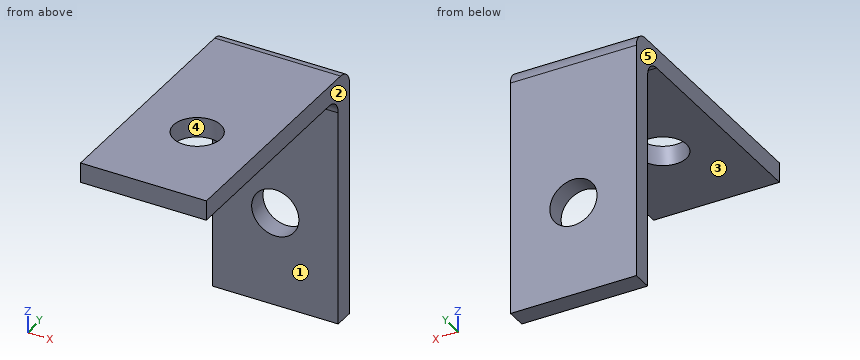
```python
from build123d import *

# Parameters (mm, degrees)
CROQUIS1_W              = 12.7
CROQUIS1_H              = 25.4
SALIENTE_EXTRUIR1_DEPTH = 2
CROQUIS2_W              = 12.7
CROQUIS2_H              = 2
SALIENTE_EXTRUIR2_DEPTH = 23.368
REDONDEO1_R             = 1.5875
CROQUIS3_R              = 2.38125
CORTAR_EXTRUIR1_DEPTH   = 26.368
CROQUIS4_R              = 2.38125
CORTAR_EXTRUIR2_DEPTH   = 2.54


with BuildPart() as part:
    # Croquis1 → Saliente-Extruir1 (new body)
    with BuildSketch(Plane(origin=(0, 0, 0), x_dir=(1, 0, 0), z_dir=(0, 1, 0))):
        Rectangle(CROQUIS1_W, CROQUIS1_H)
    extrude(amount=SALIENTE_EXTRUIR1_DEPTH)

    # Croquis2 → Saliente-Extruir2 (add)
    with BuildSketch(Plane.XZ):
        with Locations((0, 11.7)):
            Rectangle(CROQUIS2_W, CROQUIS2_H)
    extrude(amount=SALIENTE_EXTRUIR2_DEPTH)

    # Redondeo1
    redondeo1_edges = [part.edges().sort_by_distance(p)[0] for p in [
        (0, 2, 12.7),
        (0, 0, 10.7),
    ]]
    fillet(redondeo1_edges, radius=REDONDEO1_R)

    # Croquis3 → Cortar-Extruir1 (cut, through all)
    with BuildSketch(Plane(origin=(0, 2, 0), x_dir=(1, 0, 0), z_dir=(0, 1, 0))):
        with Locations((0, 3.175)):
            Circle(CROQUIS3_R)
    extrude(amount=-CORTAR_EXTRUIR1_DEPTH, mode=Mode.SUBTRACT)

    # Croquis4 → Cortar-Extruir2 (cut)
    with BuildSketch(Plane.XY.offset(12.7)):
        with Locations((0, -13.843)):
            Circle(CROQUIS4_R)
    extrude(amount=-CORTAR_EXTRUIR2_DEPTH, mode=Mode.SUBTRACT)


solid = part.part
```
Part model, mm, in its own coordinate system. Face numbers are marked on the shaded views. A direction names the side the tool comes from. Coordinates: 2 decimals unless noted, no trailing zeros. Order: outer loops, then holes, each group sorted by start corner. A loop starts at its lowest first (then second) coordinate and runs counter-clockwise, first axis right, second up. Notation, with made-up numbers: (69.5, -29) -> (106.5, -29) arc R29 ccw to (106.5, 5) -> close; hole circle Ø6 at (-11.5, -17). An arc over 180 degrees is marked (long way). Put each result on its own line as item: value. Start each with the question number.
(1) Band-saw the part on D-D (z = 2). Give the cut face in (x, y), then the cut area to 3 significant figures.
(2) Which spindle directions (+Z, -Z, +X, -X, +Y, -Y) get a long thin tool onto all of the face, cutting with end or side? Do the marked faces 1 and 2. Say none if no direction does.
(3) Mould opens along X. For the marked faces 3, 4 and 5 say: pulls with the +X half, pulls with the -X half, needs draft (parallel to the pull), parting line crosses it, or undercut.
(4) Band-saw the part on B-B (x = 4). Give the cut face in (y, z) (1 decimal).
(5) Pin check, flat tips, straight feed: pin 1 Ø6.5 at (x, z) = (-1.5, 3.5) entering from -Y; pin 2 Ø6 at (x, y) = (1, -13.5) entering from -Z. Stop position of each tip, or through.
(6) Band-saw the part on C-C (y = -5.25). Give the cut face in (x, z).
(7) Probe line 1 along Z through (x, y) = (-1.5, -18.75); line 2 along Y through (x, z) = (-1.75, 6.5); line 3 along Z through (x, y) = (0, 1.4). List the from-to ranges inside material, lowest first. Write a range as [from, to].
(8) Band-saw the part on A-A (x = 0). Give the cut face in (y, z) (1 decimal).
Determined:
1. outline: (-6.35, 0) -> (6.35, 0) -> (6.35, 2) -> (-6.35, 2) -> close
1. area: 25.4 mm²
2. face 1: -Z, +X, -X, -Y
2. face 2: +Z, -Z, +X, +Y, -Y
3. face 3: needs draft
3. face 4: undercut
3. face 5: pulls with the -X half
4. outline: (-23.4, 10.7) -> (-1.6, 10.7) arc R1.6 cw to (0, 9.1) -> (0, -12.7) -> (2, -12.7) -> (2, 11.1) arc R1.6 ccw to (0.4, 12.7) -> (-23.4, 12.7) -> close
5. pin 1: stops at y = 0
5. pin 2: stops at z = 10.7
6. outline: (-6.35, 10.7) -> (6.35, 10.7) -> (6.35, 12.7) -> (-6.35, 12.7) -> close
7. line 1: z = [10.7, 12.7]
7. line 2: y = [0, 2]
7. line 3: z = [-12.7, -5.56], [-0.79, 12.36]
8. outline: (-23.4, 10.7) -> (-16.2, 10.7) -> (-16.2, 12.7) -> (-23.4, 12.7) -> close; (-11.5, 10.7) -> (-1.6, 10.7) arc R1.6 cw to (0, 9.1) -> (0, -0.8) -> (2, -0.8) -> (2, 11.1) arc R1.6 ccw to (0.4, 12.7) -> (-11.5, 12.7) -> close; (0, -12.7) -> (2, -12.7) -> (2, -5.6) -> (0, -5.6) -> close
